The listing builds one solid part. Answer for the finished solid, in the listing's coordinates (mm). A direction names the side the tool comes from. Coordinates: 2 decimals unless noted, no trailing zeros. Loops run counter-clockwise (first coordinate to the right, second up) from the corner with the lowest first, then second, coordinate; pieces in that order, holes last. Notation, with made-up numbers: (10.5, 55.5) -> (50.5, 55.5) arc R7 ccw to (50.5, 67.5) -> close; hole circle Ø11 at (34.25, 70). An arc over 180 degrees is marked (long way). Answer in a Markdown table with one row per item.
Autodesk Inventor part; units mm, degrees
ref_plane "YZ Plane" through (0, 0, 0) normal (1, 0, 0) x (0, 1, 0)
ref_plane "XZ Plane" through (0, 0, 0) normal (0, 1, 0) x (-1, 0, 0)
ref_plane "XY Plane" through (0, 0, 0) normal (0, 0, 1) x (1, 0, 0)
sketch "Sketch1" plane through (0, 0, 0) normal (0, 0, 1) x (1, 0, 0)
  circle A0 centre (0, 0) radius 5
  dimension "d0" = 10
extrude "Extrusion1" add sketch "Sketch1" against normal blind 10
sketch "Sketch2" plane through (0, 0, 0) normal (0, 0, 1) x (1, 0, 0)
  line L0 (25, 25) -> (-25, 25)
  line L1 (-25, 25) -> (-25, -25)
  line L2 (-25, -25) -> (25, -25)
  line L3 (25, -25) -> (25, 25)
  point P0 (0, 0)
  dimension "d3" = 50
  dimension "d4" = 50
  dimension "d5" = 25
  dimension "d6" = 25
extrude "Extrusion2" add sketch "Sketch2" along normal blind 125
sketch "Sketch3" plane through (-25, 25, 0) normal (0, 1, 0) x (1, 0, 0)
  circle A0 centre (25, -100) radius 25
  line L0 (50, 0) -> (50, -125)
  line L1 (50, -125) -> (0, -125)
  line L2 (0, 0) -> (0, -125)
  circle A1 centre (25, -100) radius 5
  point P0 (25, 0)
  point P1 (25, -125)
  point P2 (50, -100)
  point P3 (0, -100)
  dimension "d9" = 10
extrude "Extrusion3" cut sketch "Sketch3" against normal through all contours L0 L1 A0 | A0 L1 L2 | A1
equation "\"d4\" = d3"
properties part number "link4"
Item 1: A cutting plane is placed at D-D, the plane x = -16.5. Determine the outline of the cut face in (y, z).
Findings below:
| item | result |
|---|---|
| outline | (-25, 0) -> (25, 0) -> (25, 118.78) -> (-25, 118.78) -> close |
Item 2: A tool of negligible diameter and unlimited length cuts with its end or side. For faces 1 (the face through (-25, 0, 49)), 2 (the face through (-1.08, -4.88, -4.93)), from which of +Z, -Z, +X, -X, +Y, -Y can it reach the whole face along a straight path? Write none if from no direction.
Findings below:
| item | result |
|---|---|
| face 1 | +Z, -Z, -X, +Y, -Y |
| face 2 | -Z |
Item 3: Find the intervals of material crossed by probe 1 along Z at (x, y) = (0, -7.5); probe 2 along Z at (x, y) = (0, 1); probe 3 along X at (y, z) = (-2.5, 100), in increasing order.
Findings below:
| item | result |
|---|---|
| probe 1 | z = 0 to 95, 105 to 125 |
| probe 2 | z = -10 to 95, 105 to 125 |
| probe 3 | x = -25 to -5, 5 to 25 |
Item 4: Flat-ended cylindrical pins translate along their axes: pin 1 Ø8 at (x, y) = (8.5, 13.5) entering from -Z; pin 2 Ø4 at (x, y) = (8.5, 14.5) entering from +Z; pin 3 Ø8 at (x, y) = (11.5, -2) entering from +Z. Find the tip coordinate at first contact, or state that the pin passes through.
Findings below:
| item | result |
|---|---|
| pin 1 | stops at z = 0 |
| pin 2 | stops at z = 124.14 |
| pin 3 | stops at z = 123.85 |
Item 5: A cutting plane is placed at A-A, the plane x = 0. Determine the outline of the cut face in (y, z).
Findings below:
| item | result |
|---|---|
| outline | (-25, 0) -> (-5, 0) -> (-5, -10) -> (5, -10) -> (5, 0) -> (25, 0) -> (25, 95) -> (-25, 95) -> close; (-25, 105) -> (25, 105) -> (25, 125) -> (-25, 125) -> close |
Item 6: Determine the mould class of faces 3 (the face through (0, 25, 62)), 4 (the face through (-1.08, 0.35, 104.88)), 5 (the face through (0, 0, -10)) for opening direction Z: +Z half, -Z half, draft (parallel to the pull), parting line (faces both ways), or undercut.
Findings below:
| item | result |
|---|---|
| face 3 | draft |
| face 4 | undercut |
| face 5 | -Z half |
Item 7: A cutting plane is placed at B-B, the plane y = 20.5. Determine the outline of the cut face in (x, z), plus the area to 3 significant figures.
Findings below:
| item | result |
|---|---|
| outline | (-25, 0) -> (25, 0) -> (25, 100) arc R25 ccw to (-25, 100) -> close; hole circle Ø10 at (0, 100) |
| area | 5,900 mm2 |
Item 8: A cutting plane is placed at C-C, the plane y = 0. Determine the outline of the cut face in (x, z).
Findings below:
| item | result |
|---|---|
| outline | (-25, 0) -> (-5, 0) -> (-5, -10) -> (5, -10) -> (5, 0) -> (25, 0) -> (25, 100) arc R25 ccw to (-25, 100) -> close; hole circle Ø10 at (0, 100) |
